Design review of the part built by this model. Coordinates are the model's own, in mm. Face numbers are marked on the shaded views. A direction names the side the tool comes from. Coordinates: 2 decimals unless noted, no trailing zeros. Write each loop counter-clockwise with the first axis right and the second up, starting at its lowest first coordinate (ties: lowest second). Pieces come first, ordered by that corner, then holes. Notation, with made-up numbers: (62, 80) -> (86, 80) arc R34 cw to (86, 117) -> close; hole circle Ø3 at (56, 77.25). An arc over 180 degrees is marked (long way). Return JSON: item names as keys, results as strings. Group by question number.
from build123d import *

# Parameters (mm, degrees)
F0_W     = 35.6
F0_H     = 30.6
F0_R     = 1.6
F1_DEPTH = 1.6
F2_R     = 12.5
F3_DEPTH = 13.1
F4_W     = 8
F4_H     = 8.6
F5_DEPTH = 9.2


with BuildPart() as f1:
    # F0 (on Front) → F1 (new body)
    with BuildSketch(Plane.XZ):
        Rectangle(F0_W, F0_H)
        with Locations((-15.2, -12.7)):
            Circle(F0_R, mode=Mode.SUBTRACT)
        with Locations((15.15, -12.65)):
            Circle(F0_R, mode=Mode.SUBTRACT)
        with Locations((-15.2, 12.7)):
            Circle(F0_R, mode=Mode.SUBTRACT)
        with Locations((15.15, 12.65)):
            Circle(F0_R, mode=Mode.SUBTRACT)
    extrude(amount=F1_DEPTH)

    # F2 (on face) → F3 (join)
    with BuildSketch(Plane.XZ.offset(1.6)):
        Circle(F2_R)
    extrude(amount=F3_DEPTH)

    # F4 (on face) → F5 (join)
    with BuildSketch(Plane(origin=(0, 0, 0), x_dir=(-1, 0, 0), z_dir=(0, 1, 0))):
        with Locations((0.2, -5)):
            Rectangle(F4_W, F4_H)
    extrude(amount=F5_DEPTH)


solid = f1.part
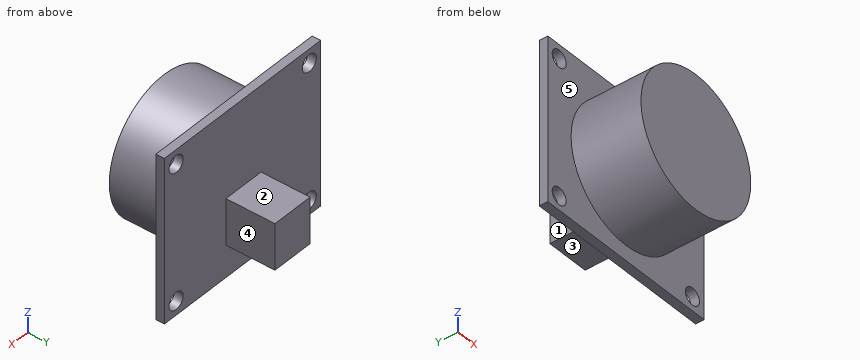
Q1. Wall thickness on L1, parallel to Z at x = 15.15, y = -0.8; L2, parallel to Z at x = -15.2, y = -1.15; L3, parallel to Y at x = -7, z = 1.5: over which ranges is each line inside the solid? List them lowest first.
Q2. For the marked faces 1, 2, 3, 4 and 5, list the 3-axis set-ups (+Z, -Z, +X, -X, +Y, -Y) from which the entire face can be reached by the end or side of a thin tool; tool diameter is ignored.
Q3. We need section B-B on z = 10. Write out the cut boundary in (x, y), plus the area to 3 significant figures.
Q4. We need section C-C on z = 13.5. Write out the cut boundary in (x, y), plus the area to 3 significant figures.
Q5. For P1, Ø3, axis at x = -2.5, y = -8.5, coming from the -Z side; P2, Ø4, axis at x = -15.2, z = 12.7, coming from the +Y side; P3, Ø7, axis at y = 4.5, z = -6.5, coming from the +X side, all flat-tipped, find the tip position at first contact; note any pin that passes through.
Q6. We need section A-A on x = -15.2. Write out the cut boundary in (y, z), plus the area to 3 significant figures.
Q7. We need section D-D on x = -3.5. Write out the cut boundary in (y, z).
Findings below:
{
 "1": {"L1": "z = -15.3 to -14.25, -11.05 to 11.05, 14.25 to 15.3", "L2": "z = -15.3 to -14.3, -11.1 to 11.1, 14.3 to 15.3", "L3": "y = -14.7 to 0"},
 "2": {"face 1": "+Z, -Z, -X, +Y", "face 2": "+Z, +X, -X, +Y", "face 3": "-Z, +X, -X, +Y", "face 4": "+Z, -Z, +X, +Y", "face 5": "-Y"},
 "3": {"outline": "(-17.8, -1.6) -> (-7.5, -1.6) -> (-7.5, -14.7) -> (7.5, -14.7) -> (7.5, -1.6) -> (17.8, -1.6) -> (17.8, 0) -> (-17.8, 0) -> close", "area": "253 mm^2"},
 "4": {"outline": "(-17.8, -1.6) -> (-16.59, -1.6) -> (-16.59, 0) -> (-17.8, 0) -> close; (-13.81, -1.6) -> (13.79, -1.6) -> (13.79, 0) -> (-13.81, 0) -> close; (16.51, -1.6) -> (17.8, -1.6) -> (17.8, 0) -> (16.51, 0) -> close", "area": "48.2 mm^2"},
 "5": {"P1": "stops at z = -12.46", "P2": "stops at y = 0", "P3": "stops at x = 3.8"},
 "6": {"outline": "(-1.6, -15.3) -> (0, -15.3) -> (0, -14.3) -> (-1.6, -14.3) -> close; (-1.6, -11.1) -> (0, -11.1) -> (0, 11.1) -> (-1.6, 11.1) -> close; (-1.6, 14.3) -> (0, 14.3) -> (0, 15.3) -> (-1.6, 15.3) -> close", "area": "38.7 mm^2"},
 "7": {"outline": "(-14.7, -12) -> (-1.6, -12) -> (-1.6, -15.3) -> (0, -15.3) -> (0, -9.3) -> (9.2, -9.3) -> (9.2, -0.7) -> (0, -0.7) -> (0, 15.3) -> (-1.6, 15.3) -> (-1.6, 12) -> (-14.7, 12) -> close"}
}
